Build history of the part. All positions in model axes, mm. A direction names the side the tool comes from. Give positions to 0.01 mm unless a question says otherwise; leave off trailing zeros. Order: outer loops, then holes, each group sorted by start corner. A loop starts at its lowest first (then second) coordinate and runs counter-clockwise, first axis right, second up. Notation, with made-up numbers: (73, 86.5) - (98, 86.5) arc R15 cw to (98, 99.5) - close; hole circle Ø10 at (77, -5.75). An arc over 180 degrees is marked (long way). Use a Markdown table: item, result.
Autodesk Inventor part; units mm, degrees
ref_plane "YZ Plane" through (0, 0, 0) normal (1, 0, 0) x (0, 1, 0)
ref_plane "XZ Plane" through (0, 0, 0) normal (0, 1, 0) x (-1, 0, 0)
ref_plane "XY Plane" through (0, 0, 0) normal (0, 0, 1) x (1, 0, 0)
sketch "Эскиз1" plane through (0, 0, 0) normal (1, 0, 0) x (0, 1, 0)
  line L0 (0, 35) -> (20.96, 35) construction
  line L1 (20.96, 35) -> (20.96, -35) construction
  line L2 (20.96, -35) -> (0, -35) construction
  line L3 (0, -35) -> (0, 35) construction
  line L4 (13, 12.5) -> (0, 12.5) construction
  line L5 (0, 12.5) -> (0, -12.5) construction
  line L6 (0, -12.5) -> (13, -12.5) construction
  line L7 (13, -12.5) -> (13, 12.5) construction
  line L8 (20.96, 17.5) -> (15.96, 17.5)
  line L9 (15.96, 17.5) -> (15.96, -17.5)
  line L10 (15.96, -17.5) -> (20.96, -17.5)
  line L11 (20.96, -17.5) -> (20.96, 17.5)
  line L12 (0, 35) -> (2, 35)
  line L13 (2, 35) -> (2, 30)
  line L14 (2, 30) -> (0, 30)
  line L15 (0, 30) -> (0, 35)
  line L16 (15.96, 17.5) -> (0, 17.5)
  line L17 (0, 30) -> (0, 17.5)
  line L18 (2, 30) -> (20.96, 17.5)
  line L19 (20.96, 0) -> (0, 0) construction
  line L20 (0, -35) -> (2, -35)
  line L21 (2, -35) -> (2, -30)
  line L22 (2, -30) -> (0, -30)
  line L23 (0, -30) -> (0, -35)
  line L24 (15.96, -17.5) -> (0, -17.5)
  line L25 (0, -30) -> (0, -17.5)
  line L26 (2, -30) -> (20.96, -17.5)
  line L27 (15.96, -17.5) -> (15.96, -17.5)
  line L28 (15.96, -17.5) -> (10.1158, -21.353)
  line L29 (15.96, -17.5) -> (22.96, -17.5) construction
  line L30 (10.1158, -21.353) -> (0, -21.353)
  line L31 (0, 17.5) -> (15.96, 6.9778)
  dimension "d0" = 20.96
  dimension "d1" = 70
  dimension "d2" = 13
  dimension "d3" = 25
  dimension "d4" = 5
  dimension "d5" = 35
  dimension "d6" = 2
  dimension "d7" = 5
  dimension "d25" = 0
  dimension "d26" = 7
extrude "Выдавливание1" add sketch "Эскиз1" along normal blind 6 contours L11 L10 L9 L8 | L8 L16 L17 L14 L18 | L9 L31 L16 | L26 L22 L25 L30 L28 L10 | L14 L15 L12 L13 | L21 L20 L23 L22
sketch "Эскиз2" plane through (0, 20.96, 17.5) normal (0, 1, 0) x (1, 0, 0)
  line L0 (0, 0) -> (6, 0)
  line L1 (3, 0) -> (3, 31) construction
  line L2 (0, 31) -> (6, 31)
  line L3 (3, 3) -> (3, 28) construction
  circle A0 centre (3, 3) radius 1.75
  circle A1 centre (3, 28) radius 1.75
  point P0 (0, 17.5)
  point P1 (3, 15.5)
  dimension "d10" = 25
  dimension "d11" = 3.5
  dimension "d12" = 3.5
extrude "Выдавливание2" cut sketch "Эскиз2" against normal blind 4
sketch "Эскиз3" plane through (0, 2, 35) normal (0, 1, 0) x (1, 0, 0)
  line L0 (0, 0) -> (6, 0) construction
  line L1 (6, 17.5) -> (6, 5)
  line L2 (0, 0) -> (6, 0) construction
  line L3 (6, 0) -> (6, 5) construction
  line L4 (6, 5) -> (0, 5) construction
  line L5 (0, 5) -> (0, 0) construction
  line L6 (6, 56.353) -> (6, 70)
  line L7 (0, 65) -> (0, 52.5)
  line L8 (6, 70) -> (0, 70) construction
  line L9 (0, 70) -> (0, 65) construction
  line L10 (0, 65) -> (6, 65) construction
  line L11 (6, 65) -> (6, 70) construction
  line L12 (0, 5) -> (0, 0) construction
  line L13 (0, 2.5) -> (6, 2.5) construction
  line L14 (3, 0) -> (3, 5) construction
  line L15 (0, 67.5) -> (6, 67.5) construction
  line L16 (3, 65) -> (3, 70) construction
  circle A0 centre (3, 2.5) radius 1.25
  circle A1 centre (3, 67.5) radius 1.25
  point P0 (0, 35)
  point P1 (6, 55.5)
  dimension "d21" = 2.5
  dimension "d22" = 2.5
extrude "Выдавливание3" cut sketch "Эскиз3" against normal blind 2
properties part number "low_part_of_extrad_system"
1) Slice it at A-A (z = 32.5). Write the cut outline in (x, y), and give its area (3 significant figures).
Computed:
| item | result |
|---|---|
| outline | (0, 0) - (1.75, 0) - (1.75, 2) - (0, 2) - close; (4.25, 0) - (6, 0) - (6, 2) - (4.25, 2) - close |
| area | 7.00 mm² |
2) Tool access for faces 1 (the flat face through (3, 16.96, -11)), 2 (the flat face through (2, 2, -34)), 3 (the flat face through (2.96, 7.87, 12.31)): list every direction of +Z, -Z, +X, -X, +Y, -Y with a clear straight run to the whole face (end or side of a thin tool).
Computed:
| item | result |
|---|---|
| face 1 | +Y |
| face 2 | -Z, +X, -X, +Y |
| face 3 | +X, -X, -Y |
3) Pin check, flat tips, straight feed: P1, Ø1, axis at x = 3.5, z = -10, coming from the +Y side; P2, Ø2, axis at x = 2, z = 8, coming from the -Y side; P3, Ø1.5, axis at x = 3, z = 31.5, coming from the +Y side. Stop position of each tip, or through.
Computed:
| item | result |
|---|---|
| P1 | stops at y = 16.96 |
| P2 | stops at y = 12.89 |
| P3 | stops at y = 2 |
4) Slice it at C-C (y = 5). Write the cut outline in (x, z), and give its area (3 significant figures).
Computed:
| item | result |
|---|---|
| outline | (0, -28.02) - (6, -28.02) - (6, -21.35) - (0, -21.35) - close; (0, 14.2) - (6, 14.2) - (6, 28.02) - (0, 28.02) - close |
| area | 123 mm² |
5) Slice it at B-B (x = 3). State how many separate pieces and enclosed holes the cut face has, and give its area (3 significant figures).
Computed:
| item | result |
|---|---|
| separate pieces | 3 |
| enclosed holes | 0 |
| area | 478 mm² |
6) Two-plate mould, pull along X, no slides. Class faces 4 (the flat face through (3, 1, -35)), 5 (the cylindrical face through (4.155, 1.014, -32.021)), 6 (the flat face through (6, 15, 8)): +X half, -X half, draft (parallel to the pull), parting line (faces both ways), or undercut.
Computed:
| item | result |
|---|---|
| face 4 | draft |
| face 5 | undercut |
| face 6 | +X half |
7) Slice it at D-D (z = -10.5). Write the cut outline in (x, y), and give its area (3 significant figures).
Computed:
| item | result |
|---|---|
| outline | (0, 15.96) - (6, 15.96) - (6, 20.96) - (4.75, 20.96) - (4.75, 16.96) - (1.25, 16.96) - (1.25, 20.96) - (0, 20.96) - close |
| area | 16.0 mm² |
8) Wall check: line 1 (X direction, y = 1.3, z = 32.5); line 2 (X direction, y = 18.75, z = -10.5); line 3 (Z direction, x = 3, y = 19.65). Give the ranges that are in metal, low to high. Write a range as from..to.
Computed:
| item | result |
|---|---|
| line 1 | x = 0..1.75, 4.25..6 |
| line 2 | x = 0..1.25, 4.75..6 |
| line 3 | z = -18.36..-12.25, -8.75..12.75, 16.25..18.36 |
